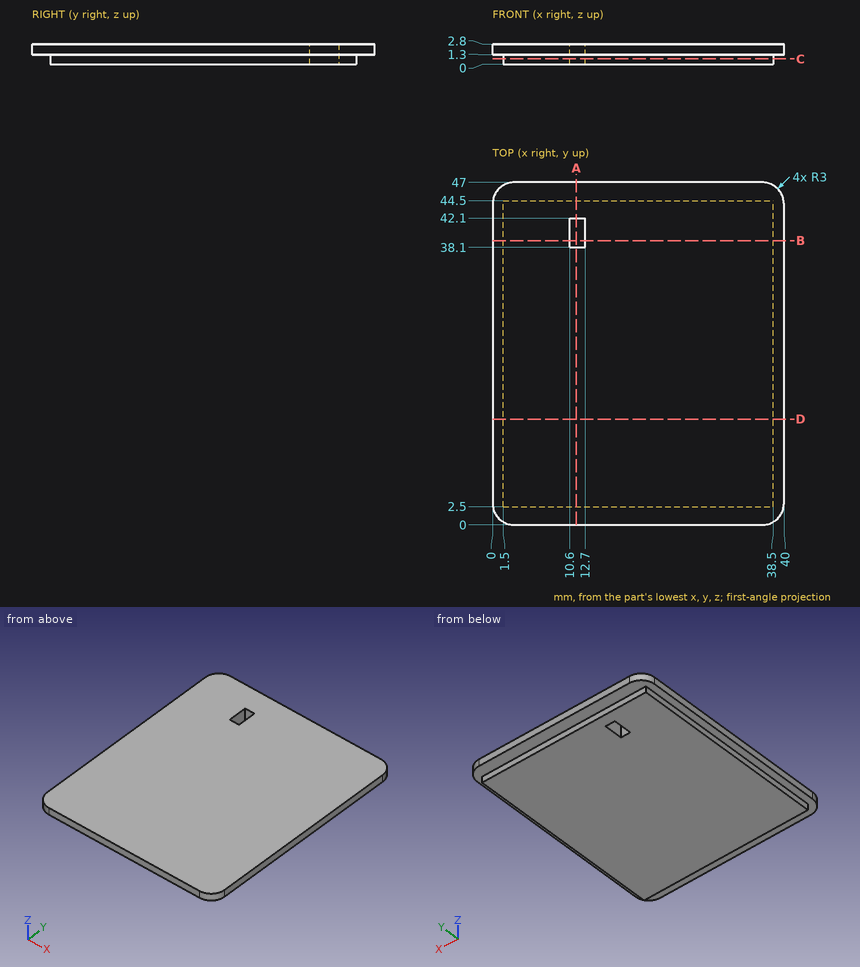
Here's the drawing with two shaded views (mm, measured from the low corner). I have some questions. Coordinates: 2 decimals unless noted, no trailing zeros. Loops run counter-clockwise (first coordinate to the right, second up) from the corner with the lowest first, then second, coordinate; pieces in that order, holes last. Notation, with made-up numbers: (-13, 51) -> (35, 51) arc R24 cw to (35, 76) -> close; hole circle Ø7 at (75.5, 53.5). An arc over 180 degrees is marked (long way). Put each result on its own line as item: value. Start each with the question number.
Q1. I want a section at B-B (y = 39). Write out the boundary of the cut face in (x, z), plus the area to 3 significant figures.
Q2. I want a section at C-C (z = 0.75). Write out the boundary of the cut face in (x, y), plus the area to 3 significant figures.
Q3. I want a section at D-D (y = 14.5). Write out the boundary of the cut face in (x, z), plus the area to 3 significant figures.
Q4. I want a section at A-A (x = 11.5). Write out the boundary of the cut face in (y, z), plus the area to 3 significant figures.
Q5. If I drill on line 1 (Y direction, x = 37.5, z = 0.6); line 2 (X direction, y = 40, z = 1.95); line 3 (X direction, y = 35, z = 0.4), over which ranges is the centre line in solid material (lowest first)? Write a range as [from, to].
Q6. I'm going to push flat-ended pins straight in: P1, Ø1.4, axis at y = 25, z = 0.5, coming from the +X side; P2, Ø0.6, axis at x = 11, z = 0.5, coming from the +Y side. Where does each tip first touch, or does it pass through?
Taken from the geometry:
1. outline: (0, 1.3) -> (1.5, 1.3) -> (1.5, 0) -> (10.6, 0) -> (10.6, 2.8) -> (0, 2.8) -> close; (12.7, 0) -> (38.5, 0) -> (38.5, 1.3) -> (40, 1.3) -> (40, 2.8) -> (12.7, 2.8) -> close
1. area: 102 mm2
2. outline: (1.5, 2.5) -> (38.5, 2.5) -> (38.5, 44.5) -> (1.5, 44.5) -> close; hole (10.6, 38.1) -> (12.7, 38.1) -> (12.7, 42.1) -> (10.6, 42.1) -> close
2. area: 1,550 mm2
3. outline: (0, 1.3) -> (1.5, 1.3) -> (1.5, 0) -> (38.5, 0) -> (38.5, 1.3) -> (40, 1.3) -> (40, 2.8) -> (0, 2.8) -> close
3. area: 108 mm2
4. outline: (0, 1.3) -> (2.5, 1.3) -> (2.5, 0) -> (38.1, 0) -> (38.1, 2.8) -> (0, 2.8) -> close; (42.1, 0) -> (44.5, 0) -> (44.5, 1.3) -> (47, 1.3) -> (47, 2.8) -> (42.1, 2.8) -> close
4. area: 114 mm2
5. line 1: y = [2.5, 44.5]
5. line 2: x = [0, 10.6], [12.7, 40]
5. line 3: x = [1.5, 38.5]
6. P1: stops at x = 38.5
6. P2: stops at y = 44.5
